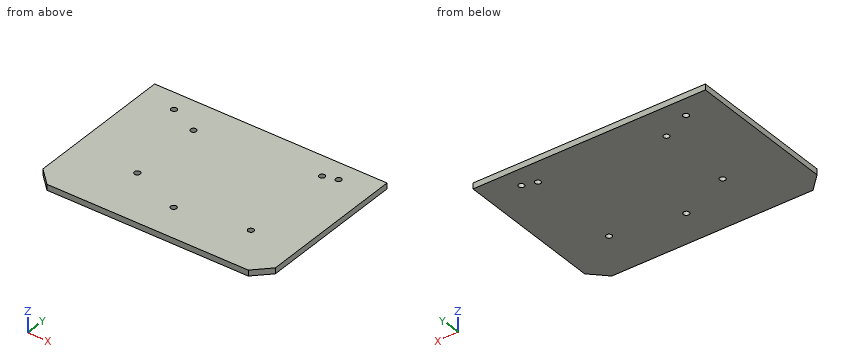
from build123d import *

# Parameters (mm, degrees)
SKETCH_1_W          = 120
SKETCH_1_H          = 85
EXTRUDE_1_DEPTH     = 3
SKETCH_2_R          = 1.5
CUT_EXTRUDE_1_DEPTH = 74.588382235
SKETCH_3_R          = 1.5
CUT_EXTRUDE_2_DEPTH = 74.588382235
CHAMFER_1_SIZE      = 8


with BuildPart() as part:
    # 草图1 → 凸台-拉伸1 (new body)
    with BuildSketch(Plane.XY):
        Rectangle(SKETCH_1_W, SKETCH_1_H)
    extrude(amount=EXTRUDE_1_DEPTH)

    # 草图2 → 切除-拉伸1 (cut, through all)
    with BuildSketch(Plane.XY.offset(3)):
        with Locations((0, -24.5)):
            Circle(SKETCH_2_R)
        with Locations((-42.5, 32.5)):
            Circle(SKETCH_2_R)
        with Locations(Location((42.5, 32.5, 0), (0, 0, 180))):
            Circle(SKETCH_2_R)
    extrude(amount=-CUT_EXTRUDE_1_DEPTH, mode=Mode.SUBTRACT)

    # 草图3 → 切除-拉伸2 (cut, through all)
    with BuildSketch(Plane.XY.offset(3)):
        with Locations((35.527993731, 30.4)):
            Circle(SKETCH_3_R)
        with Locations((-27, 25.2)):
            Circle(SKETCH_3_R)
        with Locations(Location((35.527993731, -18.7, 0), (0, 0, 180))):
            Circle(SKETCH_3_R)
        with Locations(Location((-27, -13.5, 0), (0, 0, 180))):
            Circle(SKETCH_3_R)
    extrude(amount=-CUT_EXTRUDE_2_DEPTH, mode=Mode.SUBTRACT)

    # 倒角1
    chamfer_1_edges = [part.edges().sort_by_distance(p)[0] for p in [
        (60, -42.5, 1.5),
        (-60, -42.5, 1.5),
    ]]
    chamfer(chamfer_1_edges, length=CHAMFER_1_SIZE)


solid = part.part
The model under review builds one solid part; all positions refer to its coordinate system, in mm. Round coordinates to 2 decimals unless told otherwise and drop trailing zeros. Order: outer loops, then holes, each group sorted by start corner. A loop starts at its lowest first (then second) coordinate and runs counter-clockwise, first axis right, second up. Notation, with made-up numbers: (67.5, -31) -> (116.5, -31) arc R17 ccw to (116.5, -13) -> close; hole circle Ø1 at (-5.5, 41.5). An arc over 180 degrees is marked (long way). Use CSV: the item, a comma, the result in double quotes. Start each with the question number.
(1) Consider section A-A on y = -24.5. Write out the cut boundary in (x, z), and give its area (3 significant figures).
(2) Wall thickness on probe 1 along Y at (x, z) = (42.5, 1.85): over which ranges is the line inside the solid? List them lowest first. Write a range as from..to.
(3) Consider section C-C on x = -42.5. Write out the cut boundary in (y, z).
(4) Insertion check: pin 1 (2.5 mm diameter, centred on x = 35.53, y = 30.4, fed in from -Z). The pin has a flat end and moves straight along its axis. Give the tip position at first contact, or say it passes through.
(5) Consider section B-B on x = -27. Write out the cut boundary in (y, z).
Responses:
1,outline,"(-60, 0) -> (-1.5, 0) -> (-1.5, 3) -> (-60, 3) -> close; (1.5, 0) -> (60, 0) -> (60, 3) -> (1.5, 3) -> close"
1,area,"351 mm²"
2,probe 1,"-42.5..31, 34..42.5"
3,outline,"(-42.5, 0) -> (31, 0) -> (31, 3) -> (-42.5, 3) -> close; (34, 0) -> (42.5, 0) -> (42.5, 3) -> (34, 3) -> close"
4,pin 1,"through"
5,outline,"(-42.5, 0) -> (-15, 0) -> (-15, 3) -> (-42.5, 3) -> close; (-12, 0) -> (23.7, 0) -> (23.7, 3) -> (-12, 3) -> close; (26.7, 0) -> (42.5, 0) -> (42.5, 3) -> (26.7, 3) -> close"
